Job drawing, mm, ordinate dimensions from the low corner. One solid piece. A direction names the side the tool comes from. Round coordinates to 2 decimals unless told otherwise and drop trailing zeros. Order: outer loops, then holes, each group sorted by start corner. A loop starts at its lowest first (then second) coordinate and runs counter-clockwise, first axis right, second up. Notation, with made-up numbers: (62.5, 88) - (98.5, 88) arc R22 ccw to (98.5, 108) - close; hole circle Ø8 at (15, -8). An arc over 180 degrees is marked (long way). Write each question's results on one line, items separated by ' | '. Start each with the question number.
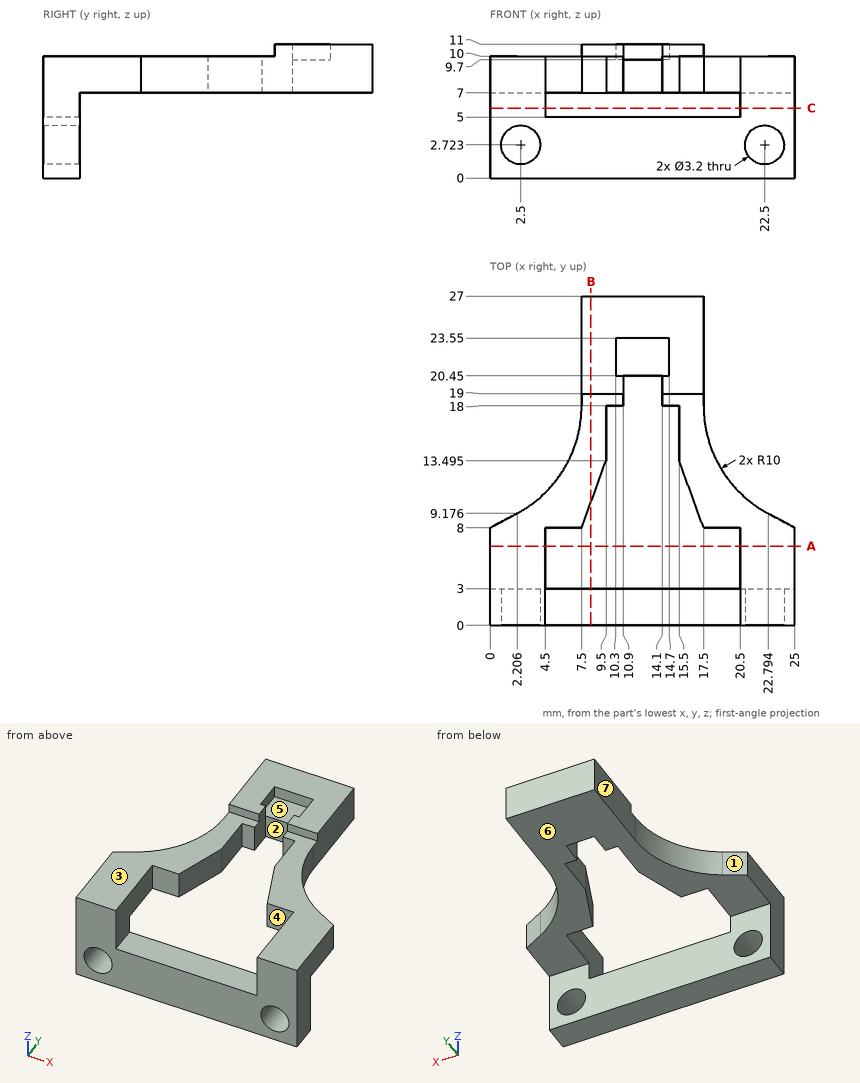
1. Cut at C-C (z = 5.75). List the corners of the cut face in (x, y), plus the area to 3 significant figures.
2. Flat gauge pins, fed straight in: pin 1 Ø1 at (y, z) = (23, 8) entering from -X; pin 2 Ø6 at (y, z) = (21.5, 5) entering from +X; pin 3 Ø5.5 at (x, y) = (4.5, 13) entering from +Z; pin 4 Ø1 at (x, y) = (7, 5) entering from +Z. Where does each tip first touch, or does it go through?
3. Wall check: line 1 (X direction, y = 3, z = 8.5); line 2 (Z direction, x = 16, y = 20.25); line 3 (Y direction, x = 1.75, z = 5.25). Give the ranges that are in metal, low to high. Write a range as from..to.
4. Cut at A-A (y = 6.5). List the corners of the cut face in (x, z).
5. 3-axis set-ups, long thin cutter, end or side, ignore diameter. For the marked faces 4, 5, 6 and 7: which of +Z, -Z, +X, -X, +Y, -Y reach the whole face in a straight line?
6. Cut at B-B (x = 8.25). List the corners of the cut face in (y, z).
7. Mould opens along X. For the marked faces 1, 2 and 3 say: pulls with the +X half, pulls with the -X half, needs draft (parallel to the pull), parting line crosses it, or undercut.
A:
1) outline: (0, 0) - (4.5, 0) - (4.5, 3) - (0, 3) - close; (20.5, 0) - (25, 0) - (25, 3) - (20.5, 3) - close | area: 27.0 mm^2
2) pin 1: stops at x = 7.5 | pin 2: stops at x = 17.5 | pin 3: stops at z = 10 | pin 4: passes through
3) line 1: x = 0..4.5, 20.5..25 | line 2: z = 7..11 | line 3: y = 0..3
4) outline: (0, 7) - (4.5, 7) - (4.5, 10) - (0, 10) - close; (20.5, 7) - (25, 7) - (25, 10) - (20.5, 10) - close
5) face 4: +Z, -Z, -Y | face 5: +Z | face 6: -Z, +X, -X, +Y | face 7: +Z, -Z, -X, +Y
6) outline: (0, 0) - (3, 0) - (3, 5) - (0, 5) - close; (10.06, 7) - (27, 7) - (27, 11) - (19, 11) - (19, 10) - (10.06, 10) - close
7) face 1: pulls with the -X half | face 2: undercut | face 3: needs draft
